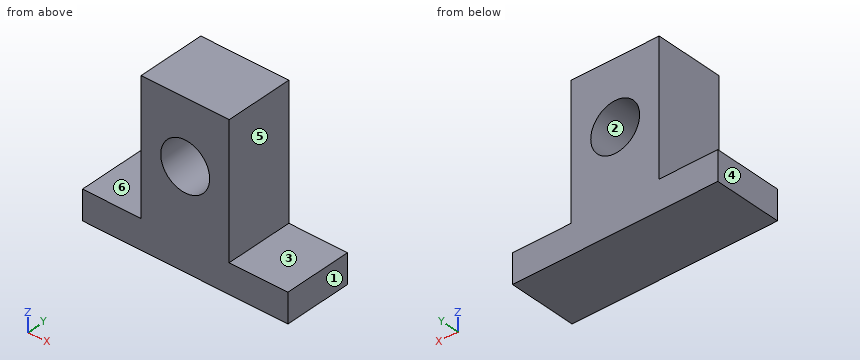
```python
from build123d import *

# Parameters (mm, degrees)
F0_W     = 42
F0_H     = 14
F1_DEPTH = 6
F2_W     = 18
F2_H     = 14
F3_DEPTH = 27
F4_R     = 5
F5_DEPTH = 14


with BuildPart() as f1:
    # F0 (on Top) → F1 (new body)
    with BuildSketch(Plane.XY):
        Rectangle(F0_W, F0_H)
    extrude(amount=F1_DEPTH)

    # F2 (on face) → F3 (join)
    with BuildSketch(Plane.XY.offset(6)):
        Rectangle(F2_W, F2_H)
    extrude(amount=F3_DEPTH)

    # F4 (on face) → F5 (cut, through all)
    with BuildSketch(Plane.XZ.offset(7)):
        with Locations((0, 20)):
            Circle(F4_R)
    extrude(amount=-F5_DEPTH, mode=Mode.SUBTRACT)


solid = f1.part
```
Geometry check sheet. Reference: the model listing, model coordinates, mm. Face numbers are marked on the shaded views. A direction names the side the tool comes from. Give positions to 0.01 mm unless a question says otherwise; leave off trailing zeros. Order: outer loops, then holes, each group sorted by start corner. A loop starts at its lowest first (then second) coordinate and runs counter-clockwise, first axis right, second up. Notation, with made-up numbers: (-27, 52.25) -> (27, 52.25) arc R14 ccw to (27, 72.25) -> close; hole circle Ø7 at (-29.75, -11). An arc over 180 degrees is marked (long way). Write each question's results on one line, items separated by ' | '. Start each with the question number.
(1) Scan lines: line 1 (Z direction, x = 0, y = 3); line 2 (Z direction, x = 17, y = -4.5); line 3 (X direction, y = 2, z = 12). Record each from-to range of solid material in increasing order.
(2) Mould release check, pull along Z, two halves, no side actions. Record for the marked faces 1, 2 and 3: pulls with the +Z half, pulls with the -Z half, needs draft (parallel to the pull), parting line crosses it, or undercut.
(3) Sectioned sample at C-C (y = -3.25). Enter the section's corners in (x, z), plus the area to 3 significant figures.
(4) Access from +Z, -Z, +X, -X, +Y, -Y to the whole of each face (thin tool, end or side, straight path). Record for the marked faces 4, 5 and 6.
(5) Gauge pin test, flat ends, axial feed: P1, Ø6, axis at y = -2, z = 29, coming from the +X side; P2, Ø5, axis at y = -2, z = 12.5, coming from the -X side; P3, Ø6, axis at x = 0, z = 20, coming from the -Y side; P4, Ø2, axis at x = 15, y = -4.5, coming from the +Z side. Record the tip position at first contact, or that the pin passes through.
(6) Sectioned sample at D-D (z = 12). Enter the section's corners in (x, y), plus the area to 3 significant figures.
(7) Sectioned sample at A-A (z = 20). Enter the section's corners in (x, y), plus the area to 3 significant figures.
(8) Sectioned sample at B-B (x = -3). Enter the section's corners in (y, z).
Answer below:
1) line 1: 0 to 15, 25 to 33 | line 2: 0 to 6 | line 3: -9 to 9
2) face 1: needs draft | face 2: undercut | face 3: pulls with the +Z half
3) outline: (-21, 0) -> (21, 0) -> (21, 6) -> (9, 6) -> (9, 33) -> (-9, 33) -> (-9, 6) -> (-21, 6) -> close; hole circle Ø10 at (0, 20) | area: 659 mm2
4) face 4: +Z, -Z, -X, +Y, -Y | face 5: +Z, +X, +Y, -Y | face 6: +Z, -X, +Y, -Y
5) P1: x = 9 | P2: x = -9 | P3: through | P4: z = 6
6) outline: (-9, -7) -> (9, -7) -> (9, 7) -> (-9, 7) -> close | area: 252 mm2
7) outline: (-9, -7) -> (-5, -7) -> (-5, 7) -> (-9, 7) -> close; (5, -7) -> (9, -7) -> (9, 7) -> (5, 7) -> close | area: 112 mm2
8) outline: (-7, 0) -> (7, 0) -> (7, 16) -> (-7, 16) -> close; (-7, 24) -> (7, 24) -> (7, 33) -> (-7, 33) -> close
